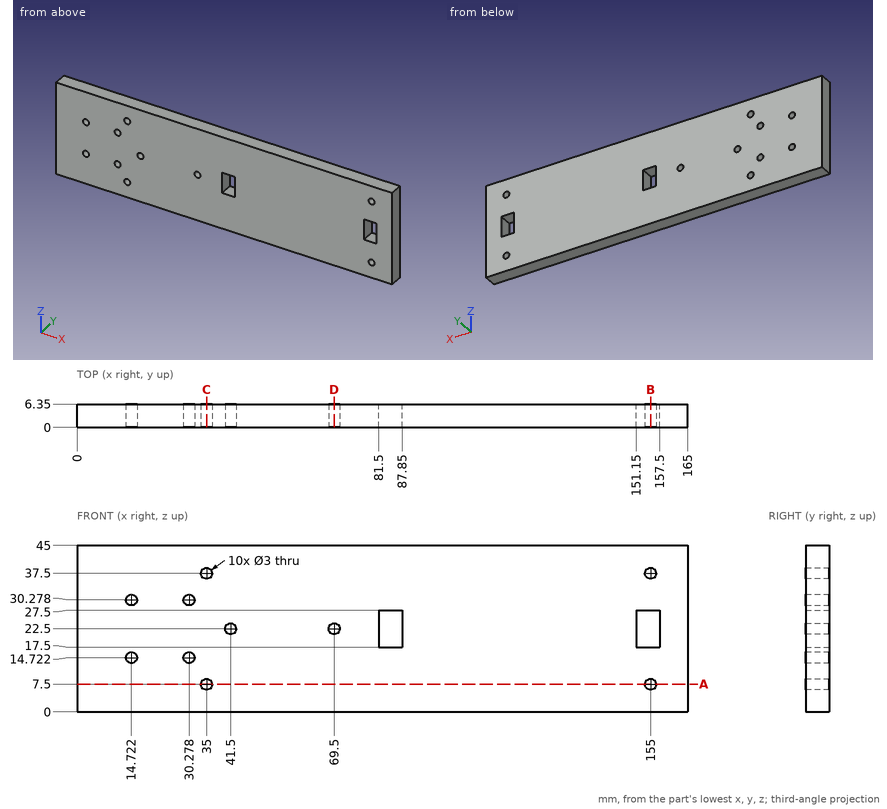
Design review of the part shown in the three views and the two pictorial views. Dimensions are in mm from the part's minimum x, y and z. Round coordinates to 2 decimals unless told otherwise and drop trailing zeros. Write each loop counter-clockwise with the first axis right and the second up, starting at its lowest first coordinate (ties: lowest second). Pieces come first, ordered by that corner, then holes.
Item 1: We need section A-A on z = 7.5. Write out the cut boundary in (x, y).
Item 2: We need section B-B on x = 155. Write out the cut boundary in (y, z), and give its area (3 significant figures).
Item 3: We need section C-C on x = 35. Write out the cut boundary in (y, z), and give its area (3 significant figures).
Item 4: For probe 1 along X at (y, z) = (3.5, 37.5); probe 2 along Z at (x, y) = (155, 2); probe 3 along X at (y, z) = (3.5, 26.5), list the stretches that pass through material, from the lowest coordinate up.
Item 5: Clearance check with a flat-ended pin moving along its axis: pin 1 Ø1.8 at (x, z) = (35, 37.5) entering from +Y. State where the tip first meets the part, or that it passes through.
Item 6: We need section D-D on x = 69.5. Write out the cut boundary in (y, z), and give its area (3 significant figures).
Returned:
1. outline: (0, 0) - (33.5, 0) - (33.5, 6.35) - (0, 6.35) - close; (36.5, 0) - (153.5, 0) - (153.5, 6.35) - (36.5, 6.35) - close; (156.5, 0) - (165, 0) - (165, 6.35) - (156.5, 6.35) - close
2. outline: (0, 0) - (6.35, 0) - (6.35, 6) - (0, 6) - close; (0, 9) - (6.35, 9) - (6.35, 17.5) - (0, 17.5) - close; (0, 27.5) - (6.35, 27.5) - (6.35, 36) - (0, 36) - close; (0, 39) - (6.35, 39) - (6.35, 45) - (0, 45) - close
2. area: 184 mm2
3. outline: (0, 0) - (6.35, 0) - (6.35, 6) - (0, 6) - close; (0, 9) - (6.35, 9) - (6.35, 36) - (0, 36) - close; (0, 39) - (6.35, 39) - (6.35, 45) - (0, 45) - close
3. area: 248 mm2
4. probe 1: x = 0 to 33.5, 36.5 to 153.5, 156.5 to 165
4. probe 2: z = 0 to 6, 9 to 17.5, 27.5 to 36, 39 to 45
4. probe 3: x = 0 to 81.5, 87.85 to 151.15, 157.5 to 165
5. pin 1: passes through
6. outline: (0, 0) - (6.35, 0) - (6.35, 21) - (0, 21) - close; (0, 24) - (6.35, 24) - (6.35, 45) - (0, 45) - close
6. area: 267 mm2
